Check sheet for the modelled part. Datum: model origin and axes. Units: mm. A direction names the side the tool comes from. Coordinates: 2 decimals unless noted, no trailing zeros. Write each loop counter-clockwise with the first axis right and the second up, starting at its lowest first coordinate (ties: lowest second). Pieces come first, ordered by that corner, then holes. Notation, with made-up numbers: (82, 26) - (110, 26) arc R25 ccw to (110, 51) - close; hole circle Ø1 at (-34, 82). An arc over 180 degrees is marked (long way). Use one line per item in the form item = value. Start each with the question number.
1. Cross-section at A-A on x = -2. Record the boundary of the cut face in (y, z).
2. Scan lines: line 1 along Y through (x, z) = (-3.25, 0); line 2 along X through (y, z) = (2, -8.25); line 3 along Y through (x, z) = (-12.75, 0). Record each from-to range of solid material in increasing order.
3. Tool access check on faces 4 (the face through (-3.8, -1.22, -0.27)), 5 (the face through (-15, 0, 0)). Record the directions out of +Z, -Z, +X, -X, +Y, -Y that give a thin tool (end or side, any length) a straight path to the whole face; none if there is none.
4. Cross-section at B-B on x = -9.75. Record the boundary of the cut face in (y, z).
5. Draft check along Y on faces 1 (the face through (0, 0, 2)), 2 (the face through (-8.12, -0.21, 0.05)), 3 (the face through (-8, 0, 10)). Enter one of: +Y half, -Y half, draft (parallel to the pull), parting line (faces both ways), or undercut.
6. Go/stop test with flat-tipped pins: pin 1 Ø1.5 at (x, y) = (-8, 5.5) entering from +Z; pin 2 Ø2 at (x, z) = (-13.5, -4.5) entering from +Y; pin 3 Ø2 at (y, z) = (0, 0) entering from +X. Record where each tip stops, or that it passes through.
```python
from build123d import *

# Parameters (mm, degrees)
M3_TAPPED_HOLE1_D     = 2.5
M3_TAPPED_HOLE1_DEPTH = 7.5
M3_TAPPED_HOLE1_TIP   = 0.751075774


with BuildPart() as part:
    # Sketch1 → Revolve1 (revolve)
    with BuildSketch(Plane.XY, mode=Mode.PRIVATE) as revolve1_sk:
        with BuildLine():
            Line((0, 0), (0, 10))
            Line((0, 10), (-15, 10))
            Line((-15, 10), (-15, 8.5))
            ThreePointArc((-15, 8.5), (-14.465142775, 6.25), (-15, 4))
            Line((-15, 4), (-15, 0))
            Line((-15, 0), (0, 0))
        make_face()
    revolve(revolve1_sk.sketch.rotate(Axis((0, 0, 0), (-1, 0, 0)), 90), axis=Axis((0, 0, 0), (-1, 0, 0)))

    # M3 Tapped Hole1
    with Locations(Plane(origin=(0, 0, 0), x_dir=(0, 0, -1), z_dir=(1, 0, 0))):
        with Locations((0, 0)):
            Hole(M3_TAPPED_HOLE1_D / 2, depth=M3_TAPPED_HOLE1_DEPTH)
            with Locations((0, 0, -(M3_TAPPED_HOLE1_DEPTH + M3_TAPPED_HOLE1_TIP / 2))):  # 118° drill point
                Cone(0, M3_TAPPED_HOLE1_D / 2, M3_TAPPED_HOLE1_TIP, mode=Mode.SUBTRACT)


solid = part.part
```
Final values:
q1.outline = circle Ø20 at (0, 0); hole circle Ø2.5 at (0, 0)
q2.line_1 = -10 to -1.25, 1.25 to 10
q2.line_2 = -14.99 to 0
q2.line_3 = -10 to 10
q3.face_4 = +X
q3.face_5 = +Z, -Z, -X, +Y, -Y
q4.outline = circle Ø20 at (0, 0)
q5.face_1 = draft
q5.face_2 = undercut
q5.face_3 = parting line
q6.pin_1 = 8.8
q6.pin_2 = 9.37
q6.pin_3 = -7.65
